For this review, take the finished solid that the model builds, in its own axes (mm). A direction names the side the tool comes from. Give positions to 0.01 mm unless a question says otherwise; leave off trailing zeros. Write each loop counter-clockwise with the first axis right and the second up, starting at its lowest first coordinate (ties: lowest second). Pieces come first, ordered by that corner, then holes.
Q1. Machinability: for faces 5 (the flat face through (0, -7.5, 4)), 6 (the flat face through (-7, -1, 8)), 7 (the flat face through (11, 5.5, 7)), 8 (the flat face through (-8, -2, 4)), which of the approach directions +Z, -Z, +X, -X, +Y, -Y give a long, thin tool a straight path to every point of the face, cutting with its end or side? Answer none if there is none.
Q2. For line 1 (X direction, y = 7.05, z = 4); line 2 (Z direction, x = 11, y = 6); line 3 (X direction, y = -5, z = 1.5), list the stretches that pass through material, from the lowest coordinate up.
Q3. We need section B-B (x = -11). Write out the cut boundary in (y, z), then the cut area to 3 significant figures.
Q4. We need section D-D (z = 6). Write out the cut boundary in (x, y).
Q5. Mouldability with a two-part tool opening along X and no side actions: class faces 1 (the flat face through (-16, 6, 4)), 2 (the flat face through (14.2, 7, 4)), 3 (the flat face through (-6, 0, 4)), 4 (the flat face through (0, -9.5, 4)) as released by +X, released by -X, zero draft, split by the parting line, or undercut.
Q6. We need section A-A (z = 4). Write out the cut boundary in (x, y).
Q7. Insertion check: P1, Ø1.9, axis at x = 11, z = 3, coming from the -Y side; P2, Ø2.5, axis at x = 2, z = 3.5, coming from the +Y side; P3, Ø2, axis at y = 1, z = 5.5, coming from the +X side. Each pin has a flat end and moves straight along its axis. Give the tip position at first contact, or say it passes through.
Q8. We need section C-C (y = -6). Write out the cut boundary in (x, z).
```python
from build123d import *

# Parameters (mm, degrees)
CROQUIS1_W              = 8
CROQUIS1_H              = 2
SALIENTE_EXTRUIR1_DEPTH = 8
CROQUIS2_R              = 2.5
CORTAR_EXTRUIR1_DEPTH   = 2
SKETCH1_W               = 8
SKETCH1_H               = 2
CUT_EXTRUDE1_DEPTH      = 1.8


with BuildPart() as part:
    # Croquis1 → Saliente-Extruir1 (new body)
    with BuildSketch(Plane.XY):
        with Locations((-12, 6.5)):
            Rectangle(CROQUIS1_W, CROQUIS1_H)
        Polygon((-6, 7.5), (-8, 7.5), (-8, 5.5), (-8, -9.5), (8, -9.5), (8, 5.5), (8, 7.5), (6, 7.5), (6, -7.5), (-6, -7.5), align=None)
        with Locations((12, 6.5)):
            Rectangle(CROQUIS1_W, CROQUIS1_H)
    extrude(amount=SALIENTE_EXTRUIR1_DEPTH)

    # Croquis2 → Cortar-Extruir1 (cut)
    with BuildSketch(Plane(origin=(0, 7.5, 0), x_dir=(1, 0, 0), z_dir=(0, 1, 0))):
        with Locations((-11, -4)):
            Circle(CROQUIS2_R)
        with Locations((11, -4)):
            Circle(CROQUIS2_R)
    extrude(amount=-CORTAR_EXTRUIR1_DEPTH, mode=Mode.SUBTRACT)

    # Sketch1 → Cut-Extrude1 (cut)
    with BuildSketch(Plane(origin=(16, 0, 0), x_dir=(0, 0, -1), z_dir=(1, 0, 0))):
        with Locations((-4, 6.5)):
            Rectangle(SKETCH1_W, SKETCH1_H)
    extrude(amount=-CUT_EXTRUDE1_DEPTH, mode=Mode.SUBTRACT)


solid = part.part
```
Computed:
1. face 5: +Z, -Z, +Y
1. face 6: +Z, +X, -X, +Y, -Y
1. face 7: +Z, -Z, +X, -Y
1. face 8: +Z, -Z, -X, -Y
2. line 1: x = -16 to -13.5, -8.5 to -6, 6 to 8.5, 13.5 to 14.2
2. line 2: z = 0 to 1.5, 6.5 to 8
2. line 3: x = -8 to -6, 6 to 8
3. outline: (5.5, 0) - (7.5, 0) - (7.5, 1.5) - (5.5, 1.5) - close; (5.5, 6.5) - (7.5, 6.5) - (7.5, 8) - (5.5, 8) - close
3. area: 6.00 mm2
4. outline: (-16, 5.5) - (-12.5, 5.5) - (-12.5, 7.5) - (-16, 7.5) - close; (-9.5, 5.5) - (-8, 5.5) - (-8, -9.5) - (8, -9.5) - (8, 5.5) - (9.5, 5.5) - (9.5, 7.5) - (6, 7.5) - (6, -7.5) - (-6, -7.5) - (-6, 7.5) - (-9.5, 7.5) - close; (12.5, 5.5) - (14.2, 5.5) - (14.2, 7.5) - (12.5, 7.5) - close
5. face 1: released by -X
5. face 2: released by +X
5. face 3: undercut
5. face 4: zero draft
6. outline: (-16, 5.5) - (-13.5, 5.5) - (-13.5, 7.5) - (-16, 7.5) - close; (-8.5, 5.5) - (-8, 5.5) - (-8, -9.5) - (8, -9.5) - (8, 5.5) - (8.5, 5.5) - (8.5, 7.5) - (6, 7.5) - (6, -7.5) - (-6, -7.5) - (-6, 7.5) - (-8.5, 7.5) - close; (13.5, 5.5) - (14.2, 5.5) - (14.2, 7.5) - (13.5, 7.5) - close
7. P1: passes through
7. P2: stops at y = -7.5
7. P3: stops at x = 8
8. outline: (-8, 0) - (-6, 0) - (-6, 8) - (-8, 8) - close; (6, 0) - (8, 0) - (8, 8) - (6, 8) - close
